Here's how the part is built. I have some questions about the finished solid (model axes, mm). A direction names the side the tool comes from. Round coordinates to 2 decimals unless told otherwise and drop trailing zeros. Loops run counter-clockwise (first coordinate to the right, second up) from the corner with the lowest first, then second, coordinate; pieces in that order, holes last. Notation, with made-up numbers: (-35.5, -22) -> (-30.5, -22) arc R31 ccw to (-30.5, 7) -> close; hole circle Ø10 at (26.25, 27.25). An arc over 180 degrees is marked (long way). Use CSV: the item, a comma, the result in double quotes. Start each with the question number.
from build123d import *

# Parameters (mm, degrees)
F1_DEPTH = 10
F3_DEPTH = 3.5
F4_R     = 2.125
F5_DEPTH = 2.5


with BuildPart() as f1:
    # F0 (on Top) → F1 (new body)
    with BuildSketch(Plane.XY):
        Polygon((-75.125, 26.563603), (-1.125, 26.563603), (-1.125, 25.063603), (-2, 25.063603), (-2, 2.063603), (-33.937408, 3.063603), (-34, 1.064582), (0, 0), (0, 40.063603), (-6, 40.063603), (-6, 28.563603), (-76.375, 28.563603), (-76.375, 20.563603), (-74.25, 20.563603), (-74.25, 25.063603), (-75.125, 25.063603), align=None)
    extrude(amount=F1_DEPTH)

    # F2 (on face) → F3 (cut)
    with BuildSketch(Plane(origin=(-6, 0, 0), x_dir=(0, -1, 0), z_dir=(-1, 0, 0))):
        Polygon((-30.563603, 2.834936), (-30.563603, 7.165064), (-34.313603, 9.330127), (-38.063603, 7.165064), (-38.063603, 2.834936), (-34.313603, 0.669873), align=None)
    extrude(amount=-F3_DEPTH, mode=Mode.SUBTRACT)

    # F4 (on face) → F5 (cut, through all)
    with BuildSketch(Plane(origin=(-2.5, 0, 0), x_dir=(0, -1, 0), z_dir=(-1, 0, 0))):
        with Locations((-34.313603, 5)):
            Circle(F4_R)
    extrude(amount=-F5_DEPTH, mode=Mode.SUBTRACT)


solid = f1.part
Q1. For faces 5 (the flat face through (-4.27, 32.46, 1.74)), 6 (the cylindrical face through (-1.27, 36, 3.71)), 7 (the flat face through (-1.125, 26, 5)), 8 (the flat face through (-41, 28.564, 5)), which set-ups out of +Z, -Z, +X, -X, +Y, -Y let a thin tool reach every point of the face, with its end or its side?
Q2. I need wall thicknesses on line 1 along X through (y, z) = (24, 5.5) (3 decimals); line 2 along Y through (x, z) = (-4.5, 1.25); line 3 along X through (y, z) = (15.5, 1.75). Which ranges of each line are inside material? Lowest first, please.
Q3. I want a section at A-A, the plane z = 5. List the corners of the cut face in (x, y) for me (3 decimals).
Q4. I want a section at C-C, the plane z = 8.25. List the corners of the cut face in (x, y) for me (3 decimals), then the cut area to 3 significant figures.
Q5. I want a section at D-D, the plane y = 4. List the corners of the cut face in (x, z) for me.
Q6. I want a section at B-B, the plane x = -33. List the corners of the cut face in (y, z) for me.
Q7. Will these pins go through, and if not, where does the flat tip stop? pin 1 Ø3 at (y, z) = (16, 3) entering from -X; pin 2 Ø2.5 at (x, z) = (-75.5, 6.5) entering from -Y; pin 3 Ø1 at (x, z) = (-3.5, 5) entering from -Y; pin 4 Ø2.5 at (y, z) = (34.31, 5) entering from -X.
Q8. If we mould it in two halves opening along Y, with no side actions, what happens to faces 1 (the flat face through (-75, 20.564, 5)), 2 (the flat face through (-21, 28, 10)), 3 (the flat face through (-2.5, 36, 3)), 4 (the flat face through (-3, 40.064, 5))? For each: pulls with the +Y half, pulls with the -Y half, needs draft (parallel to the pull), parting line crosses it, or undercut.
Values found:
1,face 5,"-X"
1,face 6,"+X, -X"
1,face 7,"+Z, -Z"
1,face 8,"+Z, -Z, -X, +Y"
2,line 1,"-76.375 to -74.25, -2 to 0"
2,line 2,"0.14 to 2.14, 26.56 to 33.31, 35.32 to 40.06"
2,line 3,"-2 to 0"
3,outline,"(-76.375, 20.564) -> (-74.25, 20.564) -> (-74.25, 25.064) -> (-75.125, 25.064) -> (-75.125, 26.564) -> (-1.125, 26.564) -> (-1.125, 25.064) -> (-2, 25.064) -> (-2, 2.064) -> (-33.937, 3.064) -> (-34, 1.065) -> (0, 0) -> (0, 32.189) -> (-2.5, 32.189) -> (-2.5, 30.564) -> (-6, 30.564) -> (-6, 28.564) -> (-76.375, 28.564) -> close; (-6, 38.064) -> (-2.5, 38.064) -> (-2.5, 36.439) -> (0, 36.439) -> (0, 40.064) -> (-6, 40.064) -> close"
4,outline,"(-76.375, 20.564) -> (-74.25, 20.564) -> (-74.25, 25.064) -> (-75.125, 25.064) -> (-75.125, 26.564) -> (-1.125, 26.564) -> (-1.125, 25.064) -> (-2, 25.064) -> (-2, 2.064) -> (-33.937, 3.064) -> (-34, 1.065) -> (0, 0) -> (0, 40.064) -> (-6, 40.064) -> (-6, 36.184) -> (-2.5, 36.184) -> (-2.5, 32.443) -> (-6, 32.443) -> (-6, 28.564) -> (-76.375, 28.564) -> close"
4,area,"336 mm2"
5,outline,"(-2, 0) -> (0, 0) -> (0, 10) -> (-2, 10) -> close"
6,outline,"(1.03, 0) -> (3.03, 0) -> (3.03, 10) -> (1.03, 10) -> close; (26.56, 0) -> (28.56, 0) -> (28.56, 10) -> (26.56, 10) -> close"
7,pin 1,"x = -2"
7,pin 2,"y = 20.56"
7,pin 3,"y = 0.09"
7,pin 4,"through"
8,face 1,"pulls with the -Y half"
8,face 2,"needs draft"
8,face 3,"undercut"
8,face 4,"pulls with the +Y half"
